from build123d import *
from build123d.topology import SkipClean

# Parameters (mm, degrees)
SKETCH_1_R          = 7
SKETCH_1_R_2        = 4
EXTRUDE_1_DEPTH     = 2
SKETCH_2_R          = 4
SKETCH_2_R_2        = 2
EXTRUDE_2_DEPTH     = 3.5
CHAMFER_1_SIZE      = 1
SKETCH_4_R          = 4
EXTRUDE_3_DEPTH     = 20
CUT_EXTRUDE_1_DEPTH = 5
CUT_EXTRUDE_2_DEPTH = 5
SKETCH_9_R          = 2.1
EXTRUDE_4_DEPTH     = 3


with BuildPart() as part:
    # 草图1 → 凸台-拉伸1 (new, symmetric)
    with BuildSketch(Plane.XY):
        Circle(SKETCH_1_R)
        Circle(SKETCH_1_R_2, mode=Mode.SUBTRACT)
    extrude(amount=EXTRUDE_1_DEPTH, both=True)

    # 草图2 → 凸台-拉伸2 (add, symmetric)
    with BuildSketch(Plane.XY):
        Circle(SKETCH_2_R)
        Circle(SKETCH_2_R_2, mode=Mode.SUBTRACT)
    extrude(amount=EXTRUDE_2_DEPTH, both=True)

    # 倒角1
    chamfer_1_edges = [part.edges().sort_by_distance(p)[0] for p in [
        (-4, 0, -3.5),
        (-4, 0, 3.5),
    ]]
    chamfer(chamfer_1_edges, length=CHAMFER_1_SIZE)

    # 草图4 → 凸台-拉伸3 (add)
    with BuildSketch(Plane(origin=(0, 25, 0), x_dir=(1, 0, 0), z_dir=(0, 1, 0))):
        with Locations(Location((0, 0, 0), (0, 0, 270))):
            Circle(SKETCH_4_R)
    extrude(amount=-EXTRUDE_3_DEPTH)

    # 草图7 → 切除-拉伸1 (cut, symmetric)
    with BuildSketch(Plane(origin=(0, 0, 0), x_dir=(0, 0, -1), z_dir=(1, 0, 0))):
        Polygon((2, 5), (4, 9), (4, 5), align=None)
        Polygon((-2, 5), (-4, 9), (-4, 5), align=None)
    extrude(amount=CUT_EXTRUDE_1_DEPTH, both=True, mode=Mode.SUBTRACT)

    # 草图8 → 切除-拉伸2 (cut, symmetric)
    with SkipClean():  # the faces are left unmerged after this step: merging them gives an invalid solid
        with BuildSketch(Plane(origin=(0, 0, 0), x_dir=(0, 0, -1), z_dir=(1, 0, 0))):
            Polygon((-2, 5), (-2, 6.08276253), (-4, 9), align=None)
            Polygon((2, 5), (2, 6.08276253), (4, 9), align=None)
        extrude(amount=CUT_EXTRUDE_2_DEPTH, both=True, mode=Mode.SUBTRACT)

    # 草图9 → 凸台-拉伸4 (add)
    with SkipClean():  # the faces are left unmerged after this step: merging them gives an invalid solid
        with BuildSketch(Plane(origin=(0, 25, 0), x_dir=(1, 0, 0), z_dir=(0, 1, 0))):
            with Locations(Location((0, 0, 0), (0, 0, 270))):
                Circle(SKETCH_9_R)
        extrude(amount=EXTRUDE_4_DEPTH)


solid = part.part
The listing builds one solid part. Answer for the finished solid, in the listing's coordinates (mm). A direction names the side the tool comes from. Give positions to 0.01 mm unless a question says otherwise; leave off trailing zeros. Loops run counter-clockwise (first coordinate to the right, second up) from the corner with the lowest first, then second, coordinate; pieces in that order, holes last. Notation, with made-up numbers: (-6.75, 39) - (13.25, 39) arc R29 cw to (13.25, 59) - close; hole circle Ø11 at (18.25, 81). An arc over 180 degrees is marked (long way). Use one line per item in the form item = value.
1. Section A-A on y = 0 is taken. Give the vertices of the cut face in (x, z).
Calculated:
outline = (-7, -2) - (-4, -2) - (-4, -2.5) - (-3, -3.5) - (-2, -3.5) - (-2, 3.5) - (-3, 3.5) - (-4, 2.5) - (-4, 2) - (-7, 2) - close; (2, -3.5) - (3, -3.5) - (4, -2.5) - (4, -2) - (7, -2) - (7, 2) - (4, 2) - (4, 2.5) - (3, 3.5) - (2, 3.5) - close
2. Which of the six approach directions +Z, -Z, +X, -X, +Y, -Y give full straight-line access (tool end or side, diameter ignored) to faces 4 (the face through (-0.048, 7.197, 2.764)), 5 (the face through (-0.867, -3.905, -2.246)), 6 (the face through (0.048, 7.197, -2.764)), 7 (the face through (-0.867, -3.905, 2.254)), 8 (the face through (0.631, 26.479, 2.003))?
Calculated:
face_4 = +Z, +X, -X
face_5 = -Z
face_6 = -Z, +X, -X
face_7 = +Z
face_8 = +Y
3. Find the intervals of material crossed by line 1 along Y through (x, z) = (0, -0.75); line 2 along Y through (x, z) = (0.5, 3); line 3 along Z through (x, y) = (-3.5, -2), in increasing order. Write a range as [from, to].
Calculated:
line_1 = [-7, -2], [2, 28]
line_2 = [-3.46, -1.94], [1.94, 3.46], [7.54, 25]
line_3 = [-2, 2]
4. Section B-B on z = 0 is taken. Give the vertices of the cut face in (x, y), then the cut area to 3 significant figures.
Calculated:
outline = (-4, 5.74) arc R7 ccw (long way) to (4, 5.74) - (4, 25) - (2.1, 25) - (2.1, 28) - (-2.1, 28) - (-2.1, 25) - (-4, 25) - close; hole circle Ø4 at (0, 0)
area = 301 mm^2
5. Section D-D on y = 25.5 is taken. Give the vertices of the cut face in (x, z), then the cut area to 3 significant figures.
Calculated:
outline = circle Ø4.2 at (0, 0)
area = 13.9 mm^2
6. Section C-C on z = -1.5 is taken. Give the vertices of the cut face in (x, y).
Calculated:
outline = (-3.71, 5.94) arc R7 ccw (long way) to (3.71, 5.94) - (3.71, 25) - (1.47, 25) - (1.47, 28) - (-1.47, 28) - (-1.47, 25) - (-3.71, 25) - close; hole circle Ø4 at (0, 0)
7. The mould has two halves that part along Y. Classify faces 1 (the face through (-1.532, 15.507, 3.695)), 2 (the face through (0, -7, 0)), 3 (the face through (0, -2, 0)): pulls with the +Y half, pulls with the -Y half, needs draft (parallel to the pull), parting line crosses it, or undercut.
Calculated:
face_1 = needs draft
face_2 = parting line crosses it
face_3 = undercut
8. Given pin 1 Ø1.2 at (x, y) = (4.5, 5.5) entering from -Z; pin 2 Ø1 at (x, y) = (4, 7) entering from +Z; pin 3 Ø6 at (x, y) = (-3.5, -2) entering from -Z, each flat-ended and moving along its own axis, determine where each tip first touches the part or whether it passes through.
Calculated:
pin_1 = -2
pin_2 = 1.94
pin_3 = -3.5
